Could you check a few things on this model? Use its own coordinates, in mm. Coordinates: 2 decimals unless noted, no trailing zeros. Order: outer loops, then holes, each group sorted by start corner. A loop starts at its lowest first (then second) coordinate and runs counter-clockwise, first axis right, second up. Notation, with made-up numbers: (-32, -29.5) - (-28, -29.5) arc R16 ccw to (-28, 0.5) - close; hole circle Ø1 at (58.25, 47.5). An arc over 180 degrees is marked (long way). One line per item, written item: value. Start each with the question number.
from build123d import *

# Parameters (mm, degrees)
F0_W        = 40.64
F0_H        = 3.0988
F1_DEPTH    = 10.16
F3_R        = 1.778
F4_T1_DEPTH = 49.7849047052
F5_DEPTH    = 25.4


# Not quite as in the source:
# - a fillet or chamfer that OpenCascade refuses, or shapes differently, is made with other operations: its cross-section is extruded or revolved along the edge and cut away or added


with BuildPart() as f1:
    # F0 (on Top) → F1 (new body)
    with BuildSketch(Plane.XY):
        with Locations((0, 1.5494)):
            Rectangle(F0_W, F0_H)
    extrude(amount=F1_DEPTH)

    # F3
    f3_edges = [f1.edges().sort_by_distance(p)[0] for p in [
        (0, 3.0988, 10.16),
    ]]
    fillet(f3_edges, radius=F3_R)

    # F4: chamfer of 1.778 on 1 edges, made by hand

    # F4_s2 → F4_t1 (cut)
    with BuildSketch(Plane.YZ.offset(-24.8924523526)):
        Polygon((1.778, 10.16), (0, 8.382), (0, 10.16), align=None)
    extrude(amount=F4_T1_DEPTH, mode=Mode.SUBTRACT)

    # F2 (on face) → F5 (cut)
    with BuildSketch(Plane.XZ):
        Polygon((-15.875, 8.5952954744), (-14.9716174209, 10.16), (-16.7783825791, 10.16), align=None)
        Polygon((-4.4531409051, 10.16), (-6.1132590949, 10.16), (-5.2832, 8.7222954744), align=None)
        Polygon((6.2853060633, 10.16), (4.3318939367, 10.16), (5.3086, 8.4682954744), align=None)
        Polygon((16.7050590949, 10.16), (15.0449409051, 10.16), (15.875, 8.7222954744), align=None)
    extrude(amount=-F5_DEPTH, mode=Mode.SUBTRACT)


solid = f1.part
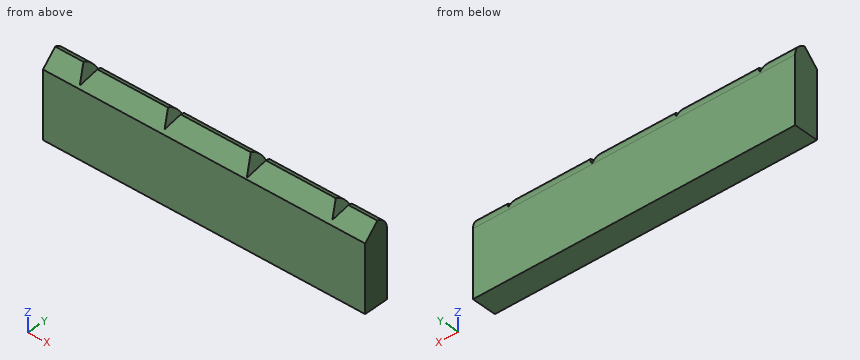
Q1. I want a section at A-A on x = -14.5. Please give me the cut outline in (y, z).
Q2. I'm going to push a flat-ended pin straight in: pin 1 (1 mm diameter, centred on x = 4, y = 1, fed in from +Z). Where does the tip first touch, or does it pass through?
Q3. If I drill on L1, parallel to Z at x = -7, y = 1.75; L2, parallel to Z at x = 13.5, y = 2.75, over which ranges is the centre line in solid material (lowest first)?
Q4. I want a section at B-B on y = 1.05. Please give me the cut outline in (x, z) (3 decimals), then the cut area to 3 significant figures.
Values follow:
1. outline: (0, 0) - (3.1, 0) - (3.1, 8.38) arc R1.78 ccw to (1.73, 10.11) - (0, 8.38) - close
2. pin 1: stops at z = 9.88
3. L1: z = 0 to 10.11
3. L2: z = 0 to 9.44
4. outline: (-20.32, 0) - (20.32, 0) - (20.32, 9.432) - (16.285, 9.432) - (15.875, 8.722) - (15.465, 9.432) - (5.865, 9.432) - (5.309, 8.468) - (4.752, 9.432) - (-4.873, 9.432) - (-5.283, 8.722) - (-5.693, 9.432) - (-15.392, 9.432) - (-15.875, 8.595) - (-16.358, 9.432) - (-20.32, 9.432) - close
4. area: 382 mm^2
